Geometry check sheet. Reference: drawing and pictorial views, mm from the part's lowest x, y, z. Give positions to 0.01 mm unless a question says otherwise; leave off trailing zeros. Order: outer loops, then holes, each group sorted by start corner. A loop starts at its lowest first (then second) coordinate and runs counter-clockwise, first axis right, second up.
Item 1: Sectioned sample at C-C on z = 9.25. Record the boundary of the cut face in (x, y), and give its area (3 significant figures).
Item 2: Sectioned sample at A-A on z = 3.75. Record the boundary of the cut face in (x, y), and give its area (3 significant figures).
Item 3: Sectioned sample at B-B on x = 10. Record the boundary of the cut face in (y, z), and give its area (3 significant figures).
Item 4: Material ranges on line 1 along X through (y, z) = (10.25, 7.25); line 2 along Y through (x, z) = (70, 2.5); line 3 along Z through (x, y) = (43.5, 6.5), recorded low to high.
Item 5: Gauge pin test, flat ends, axial feed: P1, Ø6, axis at x = 67, y = 7, coming from the -Z side; P2, Ø5, axis at x = 32.5, y = 3.5, coming from the -Z side. Record the tip position at first contact, or that the pin passes through.
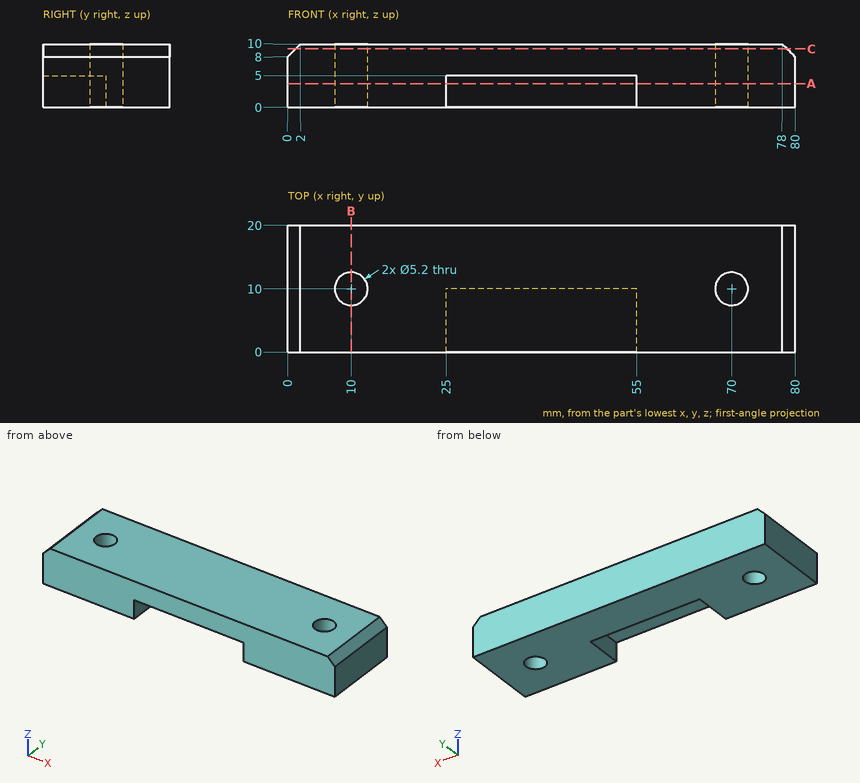
Report:
1. outline: (1.25, 0) - (78.75, 0) - (78.75, 20) - (1.25, 20) - close; hole circle Ø5.2 at (10, 10); hole circle Ø5.2 at (70, 10)
1. area: 1,510 mm2
2. outline: (0, 0) - (25, 0) - (25, 10) - (55, 10) - (55, 0) - (80, 0) - (80, 20) - (0, 20) - close; hole circle Ø5.2 at (10, 10); hole circle Ø5.2 at (70, 10)
2. area: 1,260 mm2
3. outline: (0, 0) - (7.4, 0) - (7.4, 10) - (0, 10) - close; (12.6, 0) - (20, 0) - (20, 10) - (12.6, 10) - close
3. area: 148 mm2
4. line 1: x = 0 to 7.41, 12.59 to 67.41, 72.59 to 80
4. line 2: y = 0 to 7.4, 12.6 to 20
4. line 3: z = 5 to 10
5. P1: stops at z = 0
5. P2: stops at z = 5
